Build history of the part. All positions in model axes, mm. Face numbers are marked on the shaded views. A direction names the side the tool comes from. Give positions to 0.01 mm unless a question says otherwise; leave off trailing zeros. Loops run counter-clockwise (first coordinate to the right, second up) from the corner with the lowest first, then second, coordinate; pieces in that order, holes last. Notation, with made-up numbers: M -1,10.25 L 40,10.25 A13 cw 40,29.25 Z; hole C 62.25,67.5 d10. An arc over 180 degrees is marked long. Answer as a JSON object with one key per item and string values. Group by question number.
1. Drop a flat-ended pin along its axis: pin 1 Ø3.5 at (y, z) = (11, -160.7) entering from -X. Give the stop position or say it passes through.
2. Slice it at A-A (z = -53). List the corners of the cut face in (x, y), then the cut area to 3 significant figures.
3. Slice it at B-B (x = -67). List the corners of the cut face in (y, z), then the cut area to 3 significant figures.
4. Drill centre lines: line 1 along Z through (x, y) = (-57.5, 24); line 2 along X through (y, z) = (28, -32.5); line 3 along Y through (x, z) = (-35.5, -24). Where is each one in solid material? Low to high. Write a range as [from, to].
5. 3-axis set-ups, long thin cutter, end or side, ignore diameter. For the marked faces 1 and 2: which of +Z, -Z, +X, -X, +Y, -Y reach the whole face in a straight line?
6. Mould opens along X. For the marked faces 3, 4, 5 and 6 say: released by +X, released by -X, zero draft, split by the parting line, or undercut.
7. Slice it at C-C (z = -149). List the corners of the cut face in (x, y), then the cut area to 3 significant figures.
Autodesk Inventor part; units mm, degrees
ref_plane "YZ Plane" through (0, 0, 0) normal (1, 0, 0) x (0, 1, 0)
ref_plane "XZ Plane" through (0, 0, 0) normal (0, 1, 0) x (-1, 0, 0)
ref_plane "XY Plane" through (0, 0, 0) normal (0, 0, 1) x (1, 0, 0)
sketch "servo" plane through (0, 0, 0) normal (0, 0, 1) x (1, 0, 0)
  line L0 (0, -20.0033) -> (0, 0)
  line L1 (54.4, 0) -> (54.4, -20.0033)
  line L2 (0, 0) -> (54.4, 0)
  line L3 (54.4, 0) -> (54.4, -20.0033)
  line L4 (54.4, -20.0033) -> (0, -20.0033)
  line L5 (0, -20.0033) -> (0, 0)
  circle A0 centre (3.1042, -5.0008) radius 2
  circle A1 centre (3.1042, -5.0008) radius 2
  circle A2 centre (3.1042, -15.0025) radius 2
  circle A3 centre (3.1042, -15.0025) radius 2
  circle A4 centre (51.2105, -15.0025) radius 2
  circle A5 centre (51.2105, -15.0025) radius 2
  circle A6 centre (51.2105, -5.0008) radius 2
  circle A7 centre (51.2105, -5.0008) radius 2
  line L6 (47.2, -20.0033) -> (7.2, -20.0033)
  line L7 (47.2, -20.0033) -> (7.2, -20.0033)
  line L8 (7.2, -20.0033) -> (7.2, 0)
  line L9 (7.2, 0) -> (47.2, 0)
  line L10 (47.2, 0) -> (47.2, -20.0033)
  circle A8 centre (36.7104, -10.0017) radius 2.9
  circle A9 centre (36.7104, -10.0017) radius 2.9
  point P0 (27.5156, -10.5472)
sketch "Sketch1" plane through (0, 0, 0) normal (0, 1, 0) x (-1, 0, 0)
  line L0 (0, 0) -> (120, 0)
  line L1 (120, 0) -> (120, -220)
  line L2 (120, -220) -> (0, -220)
  line L3 (0, -220) -> (0, 0)
  dimension "d0" = 120
  dimension "d1" = 220
extrude "Extrusion1" add sketch "Sketch1" along normal blind 5
sketch "Sketch3" plane through (0, 5, 0) normal (0, 1, 0) x (1, 0, 0)
  line L0 (-120, 0) -> (0, 0)
  line L1 (0, 0) -> (0, 220)
  line L2 (-120, 0) -> (0, 0)
  line L3 (0, 0) -> (0, 220)
  line L4 (0, 220) -> (-120, 220)
  line L5 (-120, 220) -> (-120, 0)
  line L6 (-115, 5) -> (-5, 5)
  line L7 (-5, 5) -> (-5, 215)
  line L8 (-5, 215) -> (-115, 215)
  line L9 (-115, 215) -> (-115, 5)
  dimension "d4" = 5
  dimension "d5" = 5
  dimension "d6" = 5
  dimension "d7" = 5
extrude "Extrusion2" add sketch "Sketch3" along normal blind 30
sketch "Sketch4" plane through (0, 0, 0) normal (1, 0, 0) x (0, 0, -1)
  line L0 (0, 0) -> (0, 35)
  line L1 (220, 0) -> (0, 0)
  line L2 (220, 0) -> (220, 35)
  line L3 (62.4, 26.0033) -> (62.4, 6)
  line L4 (8, 6) -> (8, 26.0033)
  line L5 (62.4, 6) -> (8, 6)
  line L6 (8, 6) -> (8, 26.0033)
  line L7 (8, 26.0033) -> (62.4, 26.0033)
  line L8 (62.4, 26.0033) -> (62.4, 6)
  circle A0 centre (59.2958, 11.0008) radius 2
  circle A1 centre (59.2958, 11.0008) radius 2
  circle A2 centre (59.2958, 21.0025) radius 2
  circle A3 centre (59.2958, 21.0025) radius 2
  circle A4 centre (11.1895, 21.0025) radius 2
  circle A5 centre (11.1895, 21.0025) radius 2
  circle A6 centre (11.1895, 11.0008) radius 2
  circle A7 centre (11.1895, 11.0008) radius 2
  line L9 (15.2, 26.0033) -> (55.2, 26.0033)
  line L10 (15.2, 26.0033) -> (55.2, 26.0033)
  line L11 (55.2, 26.0033) -> (55.2, 6)
  line L12 (55.2, 6) -> (15.2, 6)
  line L13 (15.2, 6) -> (15.2, 26.0033)
  circle A8 centre (25.6896, 16.0017) radius 2.9
  circle A9 centre (25.6896, 16.0017) radius 2.9
  line L14 (157.6, 6) -> (157.6, 26.0033)
  line L15 (212, 26.0033) -> (212, 6)
  line L16 (157.6, 26.0033) -> (212, 26.0033)
  line L17 (212, 26.0033) -> (212, 6)
  line L18 (212, 6) -> (157.6, 6)
  line L19 (157.6, 6) -> (157.6, 26.0033)
  circle A10 centre (160.7042, 21.0025) radius 2
  circle A11 centre (160.7042, 21.0025) radius 2
  circle A12 centre (160.7042, 11.0008) radius 2
  circle A13 centre (160.7042, 11.0008) radius 2
  circle A14 centre (208.8105, 11.0008) radius 2
  circle A15 centre (208.8105, 11.0008) radius 2
  circle A16 centre (208.8105, 21.0025) radius 2
  circle A17 centre (208.8105, 21.0025) radius 2
  line L20 (204.8, 6) -> (164.8, 6)
  line L21 (204.8, 6) -> (164.8, 6)
  line L22 (164.8, 6) -> (164.8, 26.0033)
  line L23 (164.8, 26.0033) -> (204.8, 26.0033)
  line L24 (204.8, 26.0033) -> (204.8, 6)
  circle A18 centre (194.3104, 16.0017) radius 2.9
  circle A19 centre (194.3104, 16.0017) radius 2.9
  dimension "d10" = 8
  dimension "d11" = 6
  dimension "d12" = 8
  dimension "d13" = 6
sketch "Sketch5" plane through (-120, 0, -220) normal (-1, 0, 0) x (0, 0, 1)
  line L0 (220, 0) -> (0, 0)
  line L1 (0, 0) -> (0, 35)
  line L2 (220, 0) -> (220, 35)
  line L3 (157.6, 6) -> (157.6, 26.0033)
  line L4 (212, 26.0033) -> (212, 6)
  line L5 (157.6, 26.0033) -> (212, 26.0033)
  line L6 (212, 26.0033) -> (212, 6)
  line L7 (212, 6) -> (157.6, 6)
  line L8 (157.6, 6) -> (157.6, 26.0033)
  circle A0 centre (160.7042, 21.0025) radius 2
  circle A1 centre (160.7042, 21.0025) radius 2
  circle A2 centre (160.7042, 11.0008) radius 2
  circle A3 centre (160.7042, 11.0008) radius 2
  circle A4 centre (208.8105, 11.0008) radius 2
  circle A5 centre (208.8105, 11.0008) radius 2
  circle A6 centre (208.8105, 21.0025) radius 2
  circle A7 centre (208.8105, 21.0025) radius 2
  line L9 (204.8, 6) -> (164.8, 6)
  line L10 (204.8, 6) -> (164.8, 6)
  line L11 (164.8, 6) -> (164.8, 26.0033)
  line L12 (164.8, 26.0033) -> (204.8, 26.0033)
  line L13 (204.8, 26.0033) -> (204.8, 6)
  circle A8 centre (194.3104, 16.0017) radius 2.9
  circle A9 centre (194.3104, 16.0017) radius 2.9
  line L14 (62.4, 26.0033) -> (62.4, 6)
  line L15 (8, 6) -> (8, 26.0033)
  line L16 (62.4, 6) -> (8, 6)
  line L17 (8, 6) -> (8, 26.0033)
  line L18 (8, 26.0033) -> (62.4, 26.0033)
  line L19 (62.4, 26.0033) -> (62.4, 6)
  circle A10 centre (59.2958, 11.0008) radius 2
  circle A11 centre (59.2958, 11.0008) radius 2
  circle A12 centre (59.2958, 21.0025) radius 2
  circle A13 centre (59.2958, 21.0025) radius 2
  circle A14 centre (11.1895, 21.0025) radius 2
  circle A15 centre (11.1895, 21.0025) radius 2
  circle A16 centre (11.1895, 11.0008) radius 2
  circle A17 centre (11.1895, 11.0008) radius 2
  line L20 (15.2, 26.0033) -> (55.2, 26.0033)
  line L21 (15.2, 26.0033) -> (55.2, 26.0033)
  line L22 (55.2, 26.0033) -> (55.2, 6)
  line L23 (55.2, 6) -> (15.2, 6)
  line L24 (15.2, 6) -> (15.2, 26.0033)
  circle A18 centre (25.6896, 16.0017) radius 2.9
  circle A19 centre (25.6896, 16.0017) radius 2.9
  dimension "d14" = 6
  dimension "d15" = 8
  dimension "d16" = 6
  dimension "d17" = 8
extrude "Extrusion3" cut sketch "Sketch4" against normal blind 5 contours L11 L5 L13 L7 | A0 | A2 | A4 | A6 | A8 | L22 L16 L24 L18 | A10 | A12 | A14 | A16 | A18
extrude "Extrusion4" cut sketch "Sketch5" against normal blind 5 contours L11 L5 L13 L7 | A0 | A2 | A4 | A6 | A8 | L22 L16 L24 L18 | A10 | A12 | A14 | A16 | A18
properties part number "Tronco"
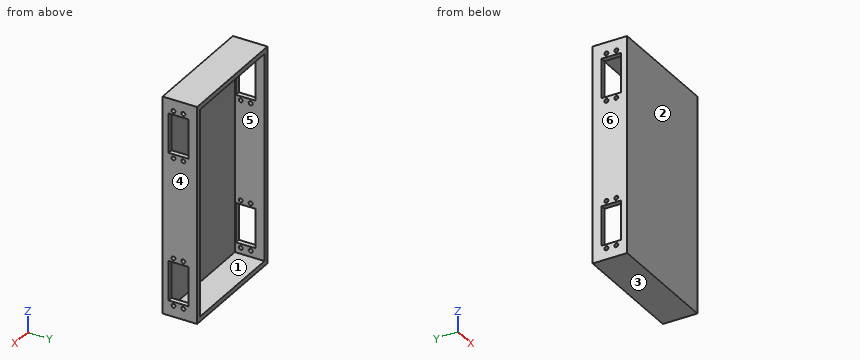
Established:
{
 "1": {"pin 1": "passes through"},
 "2": {"outline": "M -120,0 L 0,0 L 0,6 L -5,6 L -5,5 L -115,5 L -115,6 L -120,6 Z; M -120,26 L -115,26 L -115,35 L -120,35 Z; M -5,26 L 0,26 L 0,35 L -5,35 Z", "area": "700 mm^2"},
 "3": {"outline": "M 0,-220 L 35,-220 L 35,-215 L 5,-215 L 5,-5 L 35,-5 L 35,0 L 0,0 Z", "area": "1,400 mm^2"},
 "4": {"line 1": "z = [-220, -215], [-5, 0]", "line 2": "x = [-120, -115], [-5, 0]", "line 3": "y = [0, 5]"},
 "5": {"face 1": "+Y", "face 2": "+Z, -Z, +X, -X, -Y"},
 "6": {"face 3": "zero draft", "face 4": "released by +X", "face 5": "undercut", "face 6": "released by -X"},
 "7": {"outline": "M -120,0 L 0,0 L 0,35 L -5,35 L -5,5 L -115,5 L -115,35 L -120,35 Z", "area": "900 mm^2"}
}
